Source: CAD feature listing. Evaluate the final solid. Frame: model axes, mm. A direction names the side the tool comes from. Coordinates: 2 decimals unless noted, no trailing zeros. One line per question, with ' | ' between items. Start each with the question number.
Q1. Line query: line 1 (X direction, y = 77.5, z = -5.5); line 2 (Z direction, x = 0.5, y = 106); line 3 (Z direction, x = 11.5, y = 57). Output: solid intervals per line, ascending.
Q2. Access query for faces 4 (the face through (3, 250, -9)), 5 (the face through (6, 123, 0.563)), 6 (the face through (-0.001, 123, -5)). Directions: +Z, -Z, +X, -X, +Y, -Y. A direction counts if a zero-diameter tool reaches every point of the face in a straight line with its end or side. Return the directions, or none.
Q3. Draft query along X for faces 1 (the face through (18.149, 123, 2)), 2 (the face through (20.999, 123, -15)), 3 (the face through (15, 123, -20.437)). Return one class per face: +X half, -X half, draft (parallel to the pull), parting line (faces both ways), or undercut.
Q4. Contact query for flat-ended pins moving along their axis: P1, Ø3, axis at y = 181, z = -7, coming from the +X side; P2, Ø2.5, axis at x = 6.5, y = 186, coming from the +Z side; P3, Ø10, axis at y = 28.5, z = -1, coming from the -X side. Output: stop coordinate, or through.
```python
from build123d import *

# Parameters (mm, degrees)
CROQUIS1_R              = 3.645
SALIENTE_EXTRUIR1_DEPTH = 250


with BuildPart() as part:
    # Croquis1 → Saliente-Extruir1 (new body)
    with BuildSketch(Plane(origin=(0, 0, 0), x_dir=(1, 0, 0), z_dir=(0, 1, 0))):
        with BuildLine():
            Line((11.476895811, -6.713360964), (16.201895811, -6.713360964))
            Line((16.201895811, -6.713360964), (10.051895811, -0.563360964))
            Line((10.051895811, -0.563360964), (2.051895811, -0.563360964))
            Line((2.051895811, -0.563360964), (-4.098104189, -6.713360964))
            Line((-4.098104189, -6.713360964), (0.626895811, -6.713360964))
            ThreePointArc((0.626895811, -6.713360964), (2.051895811, -8.138360964), (0.626895811, -9.563360964))
            Line((0.626895811, -9.563360964), (-7.549539962, -9.536925191))
            ThreePointArc((-7.549539962, -9.536925191), (-8.538474211, -9.127295213), (-8.948104189, -8.138360964))
            Line((-8.948104189, -8.138360964), (-8.948104189, 0.011639036))
            ThreePointArc((-8.948104189, 0.011639036), (-7.549539962, 1.410203263), (-6.150975734, 0.011639036))
            Line((-6.150975734, 0.011639036), (-6.150975734, -4.713360964))
            Line((-6.150975734, -4.713360964), (-0.000975734, 1.436639036))
            Line((-0.000975734, 1.436639036), (-0.000975734, 9.436639036))
            Line((-0.000975734, 9.436639036), (-6.150975734, 15.586639036))
            Line((-6.150975734, 15.586639036), (-6.150975734, 10.861639036))
            ThreePointArc((-6.150975734, 10.861639036), (-7.575975734, 9.436639036), (-9.000975734, 10.861639036))
            Line((-9.000975734, 10.861639036), (-9.000975734, 19.011592446))
            ThreePointArc((-9.000975734, 19.011592446), (-8.583602897, 20.019219609), (-7.575975734, 20.436592446))
            Line((-7.575975734, 20.436592446), (0.574024266, 20.436592446))
            ThreePointArc((0.574024266, 20.436592446), (1.999024266, 19.011592446), (0.574024266, 17.586592446))
            Line((0.574024266, 17.586592446), (-4.150975734, 17.586592446))
            Line((-4.150975734, 17.586592446), (1.999024266, 11.436592446))
            Line((1.999024266, 11.436592446), (9.999024266, 11.436592446))
            Line((9.999024266, 11.436592446), (16.149024266, 17.586592446))
            Line((16.149024266, 17.586592446), (11.424024266, 17.586592446))
            ThreePointArc((11.424024266, 17.586592446), (9.999024266, 19.011592446), (11.424024266, 20.436592446))
            Line((11.424024266, 20.436592446), (19.574024266, 20.436592446))
            ThreePointArc((19.574024266, 20.436592446), (20.581651429, 20.019219609), (20.999024266, 19.011592446))
            Line((20.999024266, 19.011592446), (20.999024266, 10.965336131))
            ThreePointArc((20.999024266, 10.965336131), (19.574024266, 9.540336131), (18.149024266, 10.965336131))
            Line((18.149024266, 10.965336131), (18.149024266, 15.586592446))
            Line((18.149024266, 15.586592446), (11.999024266, 9.436592446))
            Line((11.999024266, 9.436592446), (11.999024266, 1.436592446))
            Line((11.999024266, 1.436592446), (18.149024266, -4.713407554))
            Line((18.149024266, -4.713407554), (18.149024266, 0.115336131))
            ThreePointArc((18.149024266, 0.115336131), (19.574024266, 1.540336131), (20.999024266, 0.115336131))
            Line((20.999024266, 0.115336131), (20.999024266, -8.138360964))
            ThreePointArc((20.999024266, -8.138360964), (20.581651429, -9.145988127), (19.574024266, -9.563360964))
            Line((19.574024266, -9.563360964), (11.476895811, -9.563360964))
            ThreePointArc((11.476895811, -9.563360964), (10.051895811, -8.138360964), (11.476895811, -6.713360964))
        make_face()
        with Locations(Location((6.051895811, 5.436639036, 0), (0, 0, 270))):
            Circle(CROQUIS1_R, mode=Mode.SUBTRACT)
    extrude(amount=SALIENTE_EXTRUIR1_DEPTH)


solid = part.part
```
Reply:
1) line 1: x = 0 to 2.41, 9.7 to 12 | line 2: z = -20.44 to -17.59, -12.94 to 2.12, 6.71 to 9.56 | line 3: z = -20.44 to -17.59, -12.94 to 2.01, 6.71 to 9.56
2) face 4: +Z, -Z, +X, -X, +Y | face 5: +Z, +Y, -Y | face 6: -X, +Y, -Y
3) face 1: undercut | face 2: +X half | face 3: draft
4) P1: stops at x = 12 | P2: stops at z = 0.56 | P3: stops at x = -8.95
